from build123d import *

# Parameters (mm, degrees)
PAD_DEPTH    = 5.7
POCKET_DEPTH = 48.9
CHAMFER_SIZE = 0.2


with BuildPart() as part:
    # Sketch → Pad (new body)
    with BuildSketch(Plane.XY):
        with BuildLine():
            Line((0, 0), (48.9, 0))
            Line((48.9, 0), (48.9, 6.3))
            ThreePointArc((48.9, 6.3), (48.548528, 7.148528), (47.7, 7.5))
            Line((45.7, 7.5), (47.7, 7.5))
            ThreePointArc((44.7, 7.5), (45.2, 7), (45.7, 7.5))
            Line((37.4, 7.5), (44.7, 7.5))
            ThreePointArc((36.4, 7.5), (36.9, 7), (37.4, 7.5))
            Line((29.1, 7.5), (36.4, 7.5))
            ThreePointArc((28.1, 7.5), (28.6, 7), (29.1, 7.5))
            Line((20.8, 7.5), (28.1, 7.5))
            ThreePointArc((19.8, 7.5), (20.3, 7), (20.8, 7.5))
            Line((12.5, 7.5), (19.8, 7.5))
            ThreePointArc((11.5, 7.5), (12, 7), (12.5, 7.5))
            Line((4.2, 7.5), (11.5, 7.5))
            ThreePointArc((3.2, 7.5), (3.7, 7), (4.2, 7.5))
            Line((1.2, 7.5), (3.2, 7.5))
            ThreePointArc((1.2, 7.5), (0.351472, 7.148528), (0, 6.3))
            Line((0, 0), (0, 6.3))
        make_face()
    extrude(amount=PAD_DEPTH)

    # Sketch001 (on Face5 of Pad) → Pocket (cut)
    with BuildSketch(Plane.YZ.offset(48.9)):
        with BuildLine():
            ThreePointArc((8.415971, 0), (5.112438, 4.453311), (0, 6.6))
            Line((0, 6.6), (8.415971, 6.6))
            Line((8.415971, 0), (8.415971, 6.6))
        make_face()
    extrude(amount=-POCKET_DEPTH, mode=Mode.SUBTRACT)

    # Chamfer
    chamfer_edges = [part.edges().sort_by_distance(p)[0] for p in [
        (48.9, 3.15, 0),
        (24.45, 0, 0),
        (0, 3.15, 0),
        (7.85, 7.5, 0),
        (16.15, 7.5, 0),
        (24.45, 7.5, 0),
        (32.75, 7.5, 0),
        (41.05, 7.5, 0),
        (0, 4.804183, 4.686015),
        (7.85, 7.5, 1.813377),
        (16.15, 7.5, 1.813377),
        (24.45, 7.5, 1.813377),
        (32.75, 7.5, 1.813377),
        (41.05, 7.5, 1.813377),
        (46.7, 7.5, 1.813377),
        (24.45, 0, 5.7),
        (48.9, 1.542589, 5.7),
        (0, 1.542589, 5.7),
        (48.9, 4.804183, 4.686015),
        (0, 0, 2.85),
        (48.9, 0, 2.85),
    ]]
    chamfer(chamfer_edges, length=CHAMFER_SIZE)


solid = part.part
The listing builds one solid part. Answer for the finished solid, in the listing's coordinates (mm). Round coordinates to 2 decimals unless told otherwise and drop trailing zeros. Write each loop counter-clockwise with the first axis right and the second up, starting at its lowest first coordinate (ties: lowest second). Pieces come first, ordered by that corner, then holes. Notation, with made-up numbers: (10, 76.5) - (38, 76.5) arc R29 cw to (38, 104.5) - close; hole circle Ø11 at (50, 70). An arc over 180 degrees is marked (long way). Use one line per item in the form item = value. Start each with the question number.
Item 1: Find the intervals of material crossed by line 1 (Y direction, x = 28.5, z = 1.3); line 2 (Y direction, x = 42, z = 3.2); line 3 (Z direction, x = 46.5, y = 7), in increasing order. Write a range as [from, to].
Item 2: A cutting plane is placed at B-B (x = 42). Write down the section's boundary in (y, z), plus the area to 3 significant figures.
Item 3: A cutting plane is placed at A-A (x = 20.3). Write down the section's boundary in (y, z).
The answers:
q1.line_1 = [0, 7.01]
q1.line_2 = [0, 6.45]
q1.line_3 = [0, 2.53]
q2.outline = (0, 0.2) - (0.2, 0) - (7.3, 0) - (7.5, 0.2) - (7.5, 1.61) - (7.39, 1.98) arc R10.49 ccw to (3.09, 5.7) - (0.2, 5.7) - (0, 5.5) - close
q2.area = 35.8 mm^2
q3.outline = (0, 0.2) - (0.2, 0) - (7, 0) - (7, 2.53) arc R10.49 ccw to (3.09, 5.7) - (0.2, 5.7) - (0, 5.5) - close
